Here's how the part is built. I have some questions about the finished solid (model axes, mm). A direction names the side the tool comes from. Round coordinates to 2 decimals unless told otherwise and drop trailing zeros. Loops run counter-clockwise (first coordinate to the right, second up) from the corner with the lowest first, then second, coordinate; pieces in that order, holes last. Notation, with made-up numbers: M 85.25,65 L 143.25,65 A20 ccw 143.25,101 Z; hole C 69.25,-25.5 d3. An arc over 180 degrees is marked long. Use a Markdown table: item, result.
```python
from build123d import *

# Parameters (mm, degrees)
SKETCH1_R           = 1.905
BOSS_EXTRUDE1_DEPTH = 3.81
FILLET1_R           = 0.635


with BuildPart() as part:
    # Sketch1 → Boss-Extrude1 (new body)
    with BuildSketch(Plane(origin=(0, 0, 0), x_dir=(1, 0, 0), z_dir=(0, 1, 0))):
        with BuildLine():
            Line((-8.89, -6.35), (-6.35, -6.35))
            Line((-6.35, -6.35), (-6.35, -12.7))
            Line((-6.35, -12.7), (6.35, -12.7))
            Line((6.35, -12.7), (6.35, -6.35))
            Line((6.35, -6.35), (8.89, -6.35))
            Line((8.89, -6.35), (3.557870234, 2.214958328))
            ThreePointArc((3.557870234, 2.214958328), (0, 4.191), (-3.557870234, 2.214958328))
            Line((-3.557870234, 2.214958328), (-8.89, -6.35))
        make_face()
        with Locations(Location((0, 0, 0), (0, 0, 90))):
            Circle(SKETCH1_R, mode=Mode.SUBTRACT)
    extrude(amount=BOSS_EXTRUDE1_DEPTH)

    # Fillet1
    fillet1_edges = [part.edges().sort_by_distance(p)[0] for p in [
        (0, 0, 12.7),
        (8.89, 1.905, 6.35),
        (6.35, 1.905, 12.7),
        (-6.35, 1.905, 12.7),
        (-8.89, 1.905, 6.35),
        (0, 3.81, 12.7),
    ]]
    fillet(fillet1_edges, radius=FILLET1_R)


solid = part.part
```
Q1. Imagine slicing it at D-D, the plane x = 2.75. Please give me the cut outline in (y, z) (3 decimals), then the cut area to 3 significant figures.
Return value:
| item | result |
|---|---|
| outline | M 0,-3.163 L 3.81,-3.163 L 3.81,12.065 A0.635 ccw 3.175,12.7 L 0.635,12.7 A0.635 ccw 0,12.065 Z |
| area | 60.3 mm^2 |
Q2. For faces 1 (the flat face through (7, 2, 6.35)), 2 (the flat face through (-6.35, 2, 9)), 3 (the flat face through (-5.89, 1.88, 1.53)), which set-ups out of +Z, -Z, +X, -X, +Y, -Y let a thin tool reach every point of the face, with its end or its side?
Return value:
| item | result |
|---|---|
| face 1 | +Z, +X, +Y, -Y |
| face 2 | +Z, -X, +Y, -Y |
| face 3 | -Z, -X, +Y, -Y |
Q3. We'd pull the mould along Z, two halves only. Please class faces 4 (the cylindrical face through (-8.3, 1.93, 6.03)), 5 (the flat face through (-7, 2, 6.35)), 6 (the flat face through (6.35, 2, 9)), 7 (the cylindrical face through (-1.89, 1.88, 0.25)): pulls with the +Z half, pulls with the -Z half, needs draft (parallel to the pull), parting line crosses it, or undercut.
Return value:
| item | result |
|---|---|
| face 4 | parting line crosses it |
| face 5 | pulls with the +Z half |
| face 6 | needs draft |
| face 7 | undercut |
Q4. Imagine slicing it at C-C, the plane y = 1.85. Please give me the cut outline in (x, z) (3 decimals), then the cut area to 3 significant figures.
Return value:
| item | result |
|---|---|
| outline | M -8.286,5.379 L -3.558,-2.215 A4.191 ccw 3.558,-2.215 L 8.286,5.379 A0.635 ccw 7.747,6.35 L 6.35,6.35 L 6.35,12.065 A0.635 ccw 5.715,12.7 L -5.715,12.7 A0.635 ccw -6.35,12.065 L -6.35,6.35 L -7.747,6.35 A0.635 ccw Z; hole C 0,0 d3.81 |
| area | 185 mm^2 |
Q5. I need wall thicknesses on line 1 (X direction, y = 1.3, z = 7.75); line 2 (Z direction, x = -0.75, y = 0.7); line 3 (X direction, y = 1.3, z = 0) (3 decimals). Which ranges of each line are inside material? Lowest first, please. Write a range as from..to.
Return value:
| item | result |
|---|---|
| line 1 | x = -6.35..6.35 |
| line 2 | z = -4.12..-1.75, 1.75..12.7 |
| line 3 | x = -4.937..-1.905, 1.905..4.937 |
Q6. Will these pins go through, and if not, where does the flat tip stop? P1, Ø1, axis at x = -5.5, y = 2, coming from the -Z side; P2, Ø1, axis at y = 1.5, z = 3, coming from the +X side; P3, Ø0.7, axis at x = -7.5, y = 2, coming from the +Z side.
Return value:
| item | result |
|---|---|
| P1 | stops at z = 0.1 |
| P2 | stops at x = 7.12 |
| P3 | stops at z = 6.35 |
Q7. Imagine slicing it at B-B, the plane z = 0. Please give me the cut outline in (x, y) (3 decimals).
Return value:
| item | result |
|---|---|
| outline | M -4.937,0 L -1.905,0 L -1.905,3.81 L -4.937,3.81 Z; M 1.905,0 L 4.937,0 L 4.937,3.81 L 1.905,3.81 Z |
Q8. Imagine slicing it at A-A, the plane x = 0. Please give me the cut outline in (y, z) (3 decimals), then the cut area to 3 significant figures.
Return value:
| item | result |
|---|---|
| outline | M 0,-4.191 L 3.81,-4.191 L 3.81,-1.905 L 0,-1.905 Z; M 0,1.905 L 3.81,1.905 L 3.81,12.065 A0.635 ccw 3.175,12.7 L 0.635,12.7 A0.635 ccw 0,12.065 Z |
| area | 49.7 mm^2 |
